Autodesk Fusion 360 part; units mm, degrees
sketch "Sketch1" plane through (0, 0, 0) normal (0, 0, 1) x (1, 0, 0)
  line L0 (0, 0) -> (40, 0)
  line L1 (40, 0) -> (40, 60)
  line L2 (40, 60) -> (0, 60)
  line L3 (0, 60) -> (0, 0)
  line L4 (20, 60) -> (20, 27.089)
  circle A0 centre (20, 40) radius 5
  line L5 (6.5, 0) -> (13.5, 0)
  line L6 (13.5, 0) -> (13.5, 25)
  line L7 (13.5, 25) -> (6.5, 25)
  line L8 (6.5, 25) -> (6.5, 0)
  line L9 (26.5, 0) -> (33.5, 0)
  line L10 (33.5, 0) -> (33.5, 25)
  line L11 (33.5, 25) -> (26.5, 25)
  line L12 (26.5, 25) -> (26.5, 0)
  line L13 (10, 25) -> (30, 25)
  line L14 (20, 25) -> (20, 0)
  line L15 (0, 16) -> (40, 16)
  line L16 (3.5, 16) -> (16.5, 16)
  line L17 (16.5, 16) -> (16.5, 9)
  line L18 (16.5, 9) -> (3.5, 9)
  line L19 (3.5, 9) -> (3.5, 16)
  line L20 (3.5, 12.5) -> (6.5, 12.5)
  line L21 (10, 9) -> (10, 0)
  line L22 (23.5, 16) -> (23.5, 9)
  line L23 (23.5, 9) -> (36.5, 9)
  line L24 (36.5, 9) -> (36.5, 16)
  dimension "d1" = 40
  dimension "d2" = 60
  dimension "d3" = 10
  dimension "d4" = 40
  dimension "d5" = 7
  dimension "d6" = 7
  dimension "d7" = 25
  dimension "d8" = 25
  dimension "d9" = 20
  dimension "d10" = 90
  dimension "d11" = 90
  dimension "d12" = 13
  dimension "d13" = 90
  dimension "d14" = 7
extrude "Extrude1" add sketch "Sketch1" along normal blind 6 contours L0 L3 L8 L15 L18 L19 | L1 L2 L3 L7 L8 L10 L11 L13 L15 L16 | L0 L6 L14 L15 L17 L18 | L0 L12 L14 L15 L22 L23 | L6 L13 L14 L15 L16 | L12 L13 L14 L15 | L0 L1 L10 L15 L23 L24
sketch "Sketch2" plane through (0, 0, 6) normal (0, 0, 1) x (-1, 0, 0)
  circle A0 centre (-20, -40) radius 5
  line L0 (-33.5, 0) -> (-40, 0)
  line L1 (-40, 0) -> (-40, -60)
  line L2 (-40, -60) -> (0, -60)
  line L3 (0, -60) -> (0, 0)
  line L4 (0, 0) -> (-6.5, 0)
  line L5 (-6.5, 0) -> (-6.5, -9)
  line L6 (-6.5, -9) -> (-3.5, -9)
  line L7 (-3.5, -9) -> (-3.5, -16)
  line L8 (-3.5, -16) -> (-6.5, -16)
  line L9 (-6.5, -16) -> (-6.5, -25)
  line L10 (-6.5, -25) -> (-13.5, -25)
  line L11 (-13.5, -25) -> (-13.5, -16)
  line L12 (-13.5, -16) -> (-16.5, -16)
  line L13 (-16.5, -16) -> (-16.5, -9)
  line L14 (-16.5, -9) -> (-13.5, -9)
  line L15 (-13.5, -9) -> (-13.5, 0)
  line L16 (-13.5, 0) -> (-26.5, 0)
  line L17 (-26.5, 0) -> (-26.5, -9)
  line L18 (-26.5, -9) -> (-23.5, -9)
  line L19 (-23.5, -9) -> (-23.5, -16)
  line L20 (-23.5, -16) -> (-26.5, -16)
  line L21 (-26.5, -16) -> (-26.5, -25)
  line L22 (-26.5, -25) -> (-33.5, -25)
  line L23 (-33.5, -25) -> (-33.5, -16)
  line L24 (-33.5, -16) -> (-36.5, -16)
  line L25 (-36.5, -16) -> (-36.5, -9)
  line L26 (-36.5, -9) -> (-33.5, -9)
  line L27 (-33.5, -9) -> (-33.5, 0)
  line L28 (0, -40) -> (-40, -40)
  line L29 (-6, -45) -> (-6, -35)
  circle A1 centre (-6, -43) radius 1.5
  circle A2 centre (-6, -37) radius 1.5
  line L30 (-6, -43) -> (-6, -37)
  line L31 (-6, -40) -> (0, -40)
  line L32 (-20, -40) -> (-20, -45)
  circle A3 centre (-34, -43) radius 1.5
  circle A4 centre (-34, -37) radius 1.5
  dimension "d17" = 6
  dimension "d18" = 3
  dimension "d19" = 3
  dimension "d20" = 6
  dimension "d21" = 90
extrude "Extrude2" cut sketch "Sketch2" against normal blind 5 contours L29 A1 L30 | L29 A1 L30 | L29 A2 L30 | L29 A2 L30 | A3 | A4
sketch "Sketch3" plane through (0, 0, 6) normal (0, 0, 1) x (-1, 0, 0)
  circle A0 centre (-6, -37) radius 1.5
  circle A1 centre (-34, -43) radius 1.5
  circle A2 centre (-6, -43) radius 1.5
  circle A3 centre (-34, -37) radius 1.5
  circle A4 centre (-20, -40) radius 5
  line L0 (-33.5, 0) -> (-40, 0)
  line L1 (-40, 0) -> (-40, -60)
  line L2 (-40, -60) -> (0, -60)
  line L3 (0, -60) -> (0, 0)
  line L4 (0, 0) -> (-6.5, 0)
  line L5 (-6.5, 0) -> (-6.5, -9)
  line L6 (-6.5, -9) -> (-3.5, -9)
  line L7 (-3.5, -9) -> (-3.5, -16)
  line L8 (-3.5, -16) -> (-6.5, -16)
  line L9 (-6.5, -16) -> (-6.5, -25)
  line L10 (-6.5, -25) -> (-13.5, -25)
  line L11 (-13.5, -25) -> (-13.5, -16)
  line L12 (-13.5, -16) -> (-16.5, -16)
  line L13 (-16.5, -16) -> (-16.5, -9)
  line L14 (-16.5, -9) -> (-13.5, -9)
  line L15 (-13.5, -9) -> (-13.5, 0)
  line L16 (-13.5, 0) -> (-26.5, 0)
  line L17 (-26.5, 0) -> (-26.5, -9)
  line L18 (-26.5, -9) -> (-23.5, -9)
  line L19 (-23.5, -9) -> (-23.5, -16)
  line L20 (-23.5, -16) -> (-26.5, -16)
  line L21 (-26.5, -16) -> (-26.5, -25)
  line L22 (-26.5, -25) -> (-33.5, -25)
  line L23 (-33.5, -25) -> (-33.5, -16)
  line L24 (-33.5, -16) -> (-36.5, -16)
  line L25 (-36.5, -16) -> (-36.5, -9)
  line L26 (-36.5, -9) -> (-33.5, -9)
  line L27 (-33.5, -9) -> (-33.5, 0)
  line L28 (0, -31) -> (-40, -31)
  line L29 (-4.5, -32.5) -> (-7.5, -32.5)
  line L30 (-7.5, -32.5) -> (-7.5, -29.5)
  line L31 (-7.5, -29.5) -> (-4.5, -29.5)
  line L32 (-4.5, -29.5) -> (-4.5, -32.5)
  line L33 (-6, -37) -> (0, -37)
  line L34 (-6, -37) -> (-6, -32.5)
  line L35 (-4.5, -31) -> (0, -31)
  line L36 (-20, -40) -> (-20, -43)
  line L37 (-35.5, -32.5) -> (-32.5, -32.5)
  line L38 (-32.5, -32.5) -> (-32.5, -29.5)
  line L39 (-35.5, -29.5) -> (-35.5, -32.5)
  line L40 (-32.5, -29.5) -> (-35.5, -29.5)
  dimension "d24" = 3
  dimension "d25" = 3
  dimension "d26" = 90
  dimension "d27" = 6
  dimension "d28" = 90
extrude "Extrude3" cut sketch "Sketch3" against normal blind 5 contours L28 L29 L30 L32 | L28 L30 L31 L32 | L28 L37 L38 L39 | L28 L38 L39 L40
fillet "Fillet1" radius 10 1 edges at (0, 60, 3)
fillet "Fillet2" radius 10 1 edges at (40, 60, 3)
extrude "Extrude4" cut 6 faces at (6.8158, 43.2169, 1) (6.1827, 37.4654, 1) (6.5, 30.5, 1) (33.5, 30.5, 1) (33.9601, 37.4654, 1) (33.2997, 43.1474, 1) along direction (0, 0, -1) blind 5
Verification items for the finished model (mm, model axes). A direction names the side the tool comes from. Coordinates: 2 decimals unless noted, no trailing zeros. Write each loop counter-clockwise with the first axis right and the second up, starting at its lowest first coordinate (ties: lowest second). Pieces come first, ordered by that corner, then holes. Notation, with made-up numbers: M -29.5,-14.5 L -22.5,-14.5 A22 ccw -22.5,-0.5 Z; hole C -1,16.5 d7. An arc over 180 degrees is marked long. Use a Markdown table: item, result.
Q1. Set-up check for faces 4 (the face through (35.5, 31, 3)), 5 (the face through (13.5, 20, 3)), 6 (the face through (20, 30, 6)): record each of +Z, -Z, +X, -X, +Y, -Y from which the full face is reachable in a straight line by a thin tool's end or side.
Reply:
| item | result |
|---|---|
| face 4 | +Z, -Z |
| face 5 | +Z, -Z, -Y |
| face 6 | +Z, +X, -X, +Y, -Y |
Q2. Draft check along X on faces 1 (the face through (40, 25, 3)), 2 (the face through (25, 9, 3)), 3 (the face through (3, 0, 3)). Enter one of: +X half, -X half, draft (parallel to the pull), parting line (faces both ways), or undercut.
Reply:
| item | result |
|---|---|
| face 1 | +X half |
| face 2 | undercut |
| face 3 | draft |
Q3. Sectioned sample at B-B, the plane y = 17. Record the boundary of the cut face in (x, z).
Reply:
| item | result |
|---|---|
| outline | M 0,0 L 6.5,0 L 6.5,6 L 0,6 Z; M 13.5,0 L 26.5,0 L 26.5,6 L 13.5,6 Z; M 33.5,0 L 40,0 L 40,6 L 33.5,6 Z |
Q4. Sectioned sample at A-A, the plane x = 20. Record the boundary of the cut face in (y, z), plus the area to 3 significant figures.
Reply:
| item | result |
|---|---|
| outline | M 0,0 L 35,0 L 35,6 L 0,6 Z; M 45,0 L 60,0 L 60,6 L 45,6 Z |
| area | 300 mm² |
Q5. Sectioned sample at D-D, the plane x = 34.5. Record the boundary of the cut face in (y, z), plus the area to 3 significant figures.
Reply:
| item | result |
|---|---|
| outline | M 0,0 L 9,0 L 9,6 L 0,6 Z; M 16,0 L 29.5,0 L 29.5,6 L 16,6 Z; M 32.5,0 L 35.59,0 L 35.59,6 L 32.5,6 Z; M 38.41,0 L 41.59,0 L 41.59,6 L 38.41,6 Z; M 44.41,0 L 58.93,0 L 58.93,6 L 44.41,6 Z |
| area | 260 mm² |
Q6. Thickness scan on line 1 (X direction, y = 19, z = 3.7); line 2 (X direction, y = 9.5, z = 4.95); line 3 (Y direction, x = 26, z = 5). Record the ranges inside material, lowest first.
Reply:
| item | result |
|---|---|
| line 1 | x = 0 to 6.5, 13.5 to 26.5, 33.5 to 40 |
| line 2 | x = 0 to 3.5, 16.5 to 23.5, 36.5 to 40 |
| line 3 | y = 0 to 9, 16 to 60 |
Q7. Go/stop test with flat-tipped pins: P1, Ø0.9, axis at x = 33.5, z = 4, coming from the +Y side; P2, Ø1, axis at x = 35.5, z = 3.5, coming from the +Y side; P3, Ø1.8, axis at x = 11, z = 3, coming from the -Y side. Record where each tip stops, or that it passes through.
Reply:
| item | result |
|---|---|
| P1 | stops at y = 59.52 |
| P2 | stops at y = 58.66 |
| P3 | stops at y = 25 |
Q8. Sectioned sample at C-C, the plane y = 43. Record the boundary of the cut face in (x, z).
Reply:
| item | result |
|---|---|
| outline | M 0,0 L 4.5,0 L 4.5,6 L 0,6 Z; M 7.5,0 L 16,0 L 16,6 L 7.5,6 Z; M 24,0 L 32.5,0 L 32.5,6 L 24,6 Z; M 35.5,0 L 40,0 L 40,6 L 35.5,6 Z |
